```python
from build123d import *

# Parameters (mm, degrees)
SKETCH1_R           = 34.925
BOSS_EXTRUDE1_DEPTH = 6.35
FILLET1_R           = 2.54
SKETCH2_R           = 2.921
CUT_EXTRUDE1_DEPTH  = 50.797929174


with BuildPart() as part:
    # Sketch1 → Boss-Extrude1 (new body)
    with BuildSketch(Plane(origin=(0, 0, 0), x_dir=(1, 0, 0), z_dir=(0, 1, 0))):
        with Locations(Location((0, 0, 0), (0, 0, 270))):
            Circle(SKETCH1_R)
        Polygon((7.918936292, 0), (3.959468146, 6.858), (-3.959468146, 6.858), (-7.918936292, 0), (-3.959468146, -6.858), (3.959468146, -6.858), align=None, mode=Mode.SUBTRACT)
    extrude(amount=BOSS_EXTRUDE1_DEPTH)

    # Fillet1
    fillet1_edges = [part.edges().sort_by_distance(p)[0] for p in [
        (0, 0, -34.925),
    ]]
    fillet(fillet1_edges, radius=FILLET1_R)

    # Sketch2 → Cut-Extrude1 (cut, through all)
    with BuildSketch(Plane(origin=(0, 6.35, 0), x_dir=(1, 0, 0), z_dir=(0, 1, 0))):
        with Locations(Location((0, 16.51, 0), (0, 0, 270))):
            Circle(SKETCH2_R)
    extrude(amount=-CUT_EXTRUDE1_DEPTH, mode=Mode.SUBTRACT)


solid = part.part
```
The listing builds one solid part. Answer for the finished solid, in the listing's coordinates (mm). A direction names the side the tool comes from. Coordinates: 2 decimals unless noted, no trailing zeros. Write each loop counter-clockwise with the first axis right and the second up, starting at its lowest first coordinate (ties: lowest second). Pieces come first, ordered by that corner, then holes. Notation, with made-up numbers: M 11.25,88.25 L 24.25,88.25 A18 cw 24.25,95.25 Z; hole C 31,28 d11. An arc over 180 degrees is marked long. Use a Markdown table: item, result. Add a question column.
1. Given P1, Ø1.5, axis at y = 2.5, z = 6, coming from the +X side; P2, Ø1.5, axis at y = 1.5, z = -7, coming from the -X side; P3, Ø5, axis at x = 10, z = 17, coming from the -Y side; P4, Ø2, axis at y = 3.5, z = -9.5, coming from the -X side, each flat-ended and moving along its own axis, determine where each tip first touches the part or whether it passes through.
2. For a pull along X with two mould halves and no side action, classify faces 1 (the flat face through (0, 0, -8)), 2 (the cylindrical face through (-34.094, 4.418, -7.571)), 3 (the flat face through (-5.9, 3.1, -3.5)) as +X half, -X half, draft (parallel to the pull), parting line (faces both ways), or undercut.
3. Section B-B (x = 0) is taken. Give the vertices of the cut face in (y, z) (3 decimals), plus the area to 3 significant figures.
4. Straight lines are drawn through the part: line 1 along X through (y, z) = (3, -16.51); line 2 along Z through (x, y) = (-7.5, 5); line 3 along Z through (x, y) = (3.5, 0.75). For each, find the intervals that lie inside material, in ascending order. Write a range as [from, to].
5. Section A-A (y = 4.25) is taken. Give the vertices of the cut face in (x, z) (3 decimals), plus the area to 3 significant figures.
6. Which of the six approach directions +Z, -Z, +X, -X, +Y, -Y give full straight-line access (tool end or side, diameter ignored) to faces 4 (the flat face through (0.5, 6.35, 7.3)), 5 (the flat face through (0, 3, -6.858))?
Data:
| question | item | result |
|---|---|---|
| 1 | P1 | stops at x = 34.53 |
| 1 | P2 | stops at x = -34.27 |
| 1 | P3 | stops at y = 0 |
| 1 | P4 | stops at x = -33.87 |
| 2 | face 1 | draft |
| 2 | face 2 | parting line |
| 2 | face 3 | undercut |
| 3 | outline | M 0,-32.385 A2.54 ccw 2.54,-34.925 L 6.35,-34.925 L 6.35,-19.431 L 0,-19.431 Z; M 0,-13.589 L 6.35,-13.589 L 6.35,-6.858 L 0,-6.858 Z; M 0,6.858 L 6.35,6.858 L 6.35,34.925 L 2.54,34.925 A2.54 ccw 0,32.385 Z |
| 3 | area | 317 mm2 |
| 4 | line 1 | x = [-30.78, -2.92], [2.92, 30.78] |
| 4 | line 2 | z = [-34.11, -0.73], [0.73, 34.11] |
| 4 | line 3 | z = [-34.01, -6.86], [6.86, 34.01] |
| 5 | outline | C 0,0 d69.85; hole M -7.919,0 L -3.959,-6.858 L 3.959,-6.858 L 7.919,0 L 3.959,6.858 L -3.959,6.858 Z; hole C 0,-16.51 d5.842 |
| 5 | area | 3,640 mm2 |
| 6 | face 4 | +Z, -Z, +X, -X, +Y |
| 6 | face 5 | +Y, -Y |
